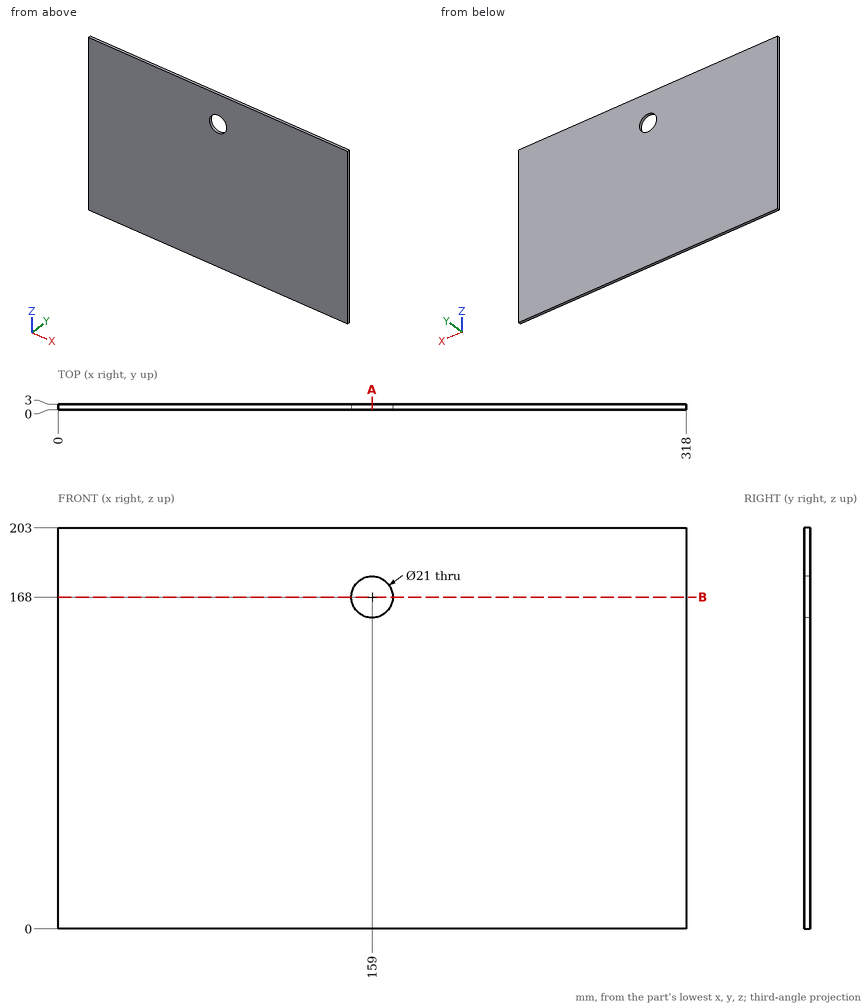
Geometry: see drawing. Coordinates: mm, zero at the bounding-box minimum. Round coordinates to 2 decimals unless told otherwise and drop trailing zeros. Write each loop counter-clockwise with the first axis right and the second up, starting at its lowest first coordinate (ties: lowest second). Pieces come first, ordered by that corner, then holes.
Item 1: Section query B-B (z = 168). Return loops of the section in (x, y), plus the area to 3 significant figures.
Item 2: Section query A-A (x = 159). Return loops of the section in (y, z), plus the area to 3 significant figures.
Item 3: Material intervals for L1, parallel to Z at x = 159, y = 1.15; L2, parallel to X at y = 1.2, z = 161.5; L3, parallel to X at y = 1.85, z = 159, sorted ascending.
Completed:
1. outline: (0, 0) - (148.5, 0) - (148.5, 3) - (0, 3) - close; (169.5, 0) - (318, 0) - (318, 3) - (169.5, 3) - close
1. area: 891 mm2
2. outline: (0, 0) - (3, 0) - (3, 157.5) - (0, 157.5) - close; (0, 178.5) - (3, 178.5) - (3, 203) - (0, 203) - close
2. area: 546 mm2
3. L1: z = 0 to 157.5, 178.5 to 203
3. L2: x = 0 to 150.75, 167.25 to 318
3. L3: x = 0 to 153.59, 164.41 to 318
